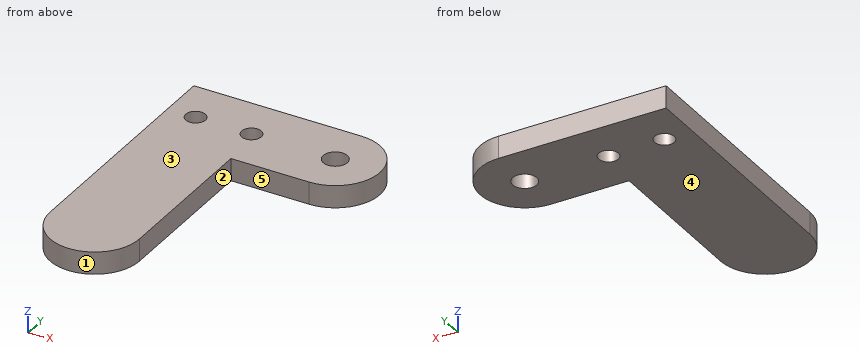
from build123d import *

# Parameters (mm, degrees)
BOSS_EXTRUDE1_DEPTH  = 5.08
M5_CLEARANCE_HOLE1_D = 5.5
M4_CLEARANCE_HOLE1_D = 4.5


with BuildPart() as part:
    # Sketch1 → Boss-Extrude1 (new body)
    with BuildSketch(Plane.XY):
        with BuildLine():
            Line((0, 10.16), (0, -10.16))
            Line((0, -10.16), (0, -45.72))
            ThreePointArc((0, -45.72), (10.16, -55.88), (20.32, -45.72))
            Line((20.32, -45.72), (20.32, -10.16))
            Line((20.32, -10.16), (38.1, -10.16))
            ThreePointArc((38.1, -10.16), (48.26, 0), (38.1, 10.16))
            Line((38.1, 10.16), (0, 10.16))
        make_face()
    extrude(amount=BOSS_EXTRUDE1_DEPTH)

    # M5 Clearance Hole1 (through all)
    with Locations(Plane.XY.offset(5.08)):
        with Locations((38.1, 0)):
            Hole(M5_CLEARANCE_HOLE1_D / 2)

    # M4 Clearance Hole1 (through all)
    with Locations(Plane.XY.offset(5.08)):
        with Locations((19.05, -0.016311357), (6.35, -0.016311357)):
            Hole(M4_CLEARANCE_HOLE1_D / 2)


solid = part.part
Can you work these out from the model? Positions are in its coordinate system, mm. Face numbers are marked on the shaded views. A direction names the side the tool comes from. Round coordinates to 2 decimals unless told otherwise and drop trailing zeros. Order: outer loops, then holes, each group sorted by start corner. A loop starts at its lowest first (then second) coordinate and runs counter-clockwise, first axis right, second up. Notation, with made-up numbers: M -17.75,-3 L 28.25,-3 A12 cw 28.25,11 Z; hole C 74,72.25 d8. An arc over 180 degrees is marked long. Use a Markdown table: item, result.
1) On a 3-axis mill with a long thin cutter (end or side, diameter ignored), from which of +Z, -Z, +X, -X, +Y, -Y can I reach the whole of each face in a straight line? I mean the marked faces 4 and 5. Say none if no direction works.
Geometry says:
| item | result |
|---|---|
| face 4 | -Z, +X, -X, +Y, -Y |
| face 5 | +Z, -Z, +X, -Y |
2) Imagine slicing it at B-B (x = 19.05). List the corners of the cut face in (y, z) for me.
Geometry says:
| item | result |
|---|---|
| outline | M -50.64,0 L -2.27,0 L -2.27,5.08 L -50.64,5.08 Z; M 2.23,0 L 10.16,0 L 10.16,5.08 L 2.23,5.08 Z |
3) If I drill on line 1 along Y through (x, z) = (38.1, 3.5); line 2 along X through (y, z) = (-23.5, 3); line 3 along Y through (x, z) = (39, 1.15), over which ranges is the centre line in solid material (lowest first)?
Geometry says:
| item | result |
|---|---|
| line 1 | y = -10.16 to -2.75, 2.75 to 10.16 |
| line 2 | x = 0 to 20.32 |
| line 3 | y = -10.12 to -2.6, 2.6 to 10.12 |
4) If we mould it in two halves opening along X, with no side actions, what happens to the marked faces 1, 2 and 3? For each: +X half, -X half, draft (parallel to the pull), parting line (faces both ways), or undercut.
Geometry says:
| item | result |
|---|---|
| face 1 | parting line |
| face 2 | +X half |
| face 3 | draft |
5) Imagine slicing it at C-C (y = 1.5). List the corners of the cut face in (x, z) for me.
Geometry says:
| item | result |
|---|---|
| outline | M 0,0 L 4.69,0 L 4.69,5.08 L 0,5.08 Z; M 8.01,0 L 17.39,0 L 17.39,5.08 L 8.01,5.08 Z; M 20.71,0 L 35.8,0 L 35.8,5.08 L 20.71,5.08 Z; M 40.4,0 L 48.15,0 L 48.15,5.08 L 40.4,5.08 Z |
6) Imagine slicing it at D-D (y = -35.5). List the corners of the cut face in (x, z) for me, then the cut area to 3 significant figures.
Geometry says:
| item | result |
|---|---|
| outline | M 0,0 L 20.32,0 L 20.32,5.08 L 0,5.08 Z |
| area | 103 mm² |
7) I'm going to push a flat-ended pin straight in: P1, Ø3, axis at x = 37.5, z = 3, coming from the -Y side. Where does the tip first touch, or does it pass through?
Geometry says:
| item | result |
|---|---|
| P1 | stops at y = -10.16 |
8) Imagine slicing it at A-A (z = 1.5). List the corners of the cut face in (x, y) for me, then the cut area to 3 significant figures.
Geometry says:
| item | result |
|---|---|
| outline | M 0,-45.72 A10.16 ccw 20.32,-45.72 L 20.32,-10.16 L 38.1,-10.16 A10.16 ccw 38.1,10.16 L 0,10.16 Z; hole C 6.35,-0.02 d4.5; hole C 19.05,-0.02 d4.5; hole C 38.1,0 d5.5 |
| area | 1,770 mm² |
